CAD build for the part. Positions are in the model's coordinates, mm. Face numbers are marked on the shaded views. A direction names the side the tool comes from. Round coordinates to 2 decimals unless told otherwise and drop trailing zeros. Order: outer loops, then holes, each group sorted by start corner. A loop starts at its lowest first (then second) coordinate and runs counter-clockwise, first axis right, second up.
```python
from build123d import *

# Parameters (mm, degrees)
SKETCH_R     = 3.5
SKETCH_R_2   = 3.25
PAD_DEPTH    = 2.8
SKETCH001_R  = 4.9
PAD001_DEPTH = 5.7
PAD002_DEPTH = 11.8
SKETCH004_W  = 6.6
SKETCH004_H  = 10
PAD003_DEPTH = 6.4
SKETCH005_W  = 10
SKETCH005_H  = 6.6
SKETCH006_W  = 10
SKETCH006_H  = 5.3


with BuildPart() as part:
    # Sketch → Pad (new body)
    with BuildSketch(Plane.XZ):
        Circle(SKETCH_R)
        Circle(SKETCH_R_2, mode=Mode.SUBTRACT)
    extrude(amount=PAD_DEPTH)

    # Sketch001 (on Face4 of Pad) → Pad001 (join)
    with BuildSketch(Plane.XZ.offset(2.8)):
        Circle(SKETCH001_R)
    extrude(amount=PAD001_DEPTH)

    # Sketch002 → AdditiveLoft section 0
    with BuildSketch(Plane.XZ.offset(8.5)):
        with BuildLine():
            Line((-5.5, 2.668195), (-5.5, -2.668195))
            ThreePointArc((-5.5, -2.668195), (-4.568071, -4.918071), (-2.318195, -5.85))
            Line((-2.318195, -5.85), (2.318195, -5.85))
            ThreePointArc((2.318195, -5.85), (4.568071, -4.918071), (5.5, -2.668195))
            Line((5.5, -2.668195), (5.5, 2.668195))
            ThreePointArc((5.5, 2.668195), (4.568071, 4.918071), (2.318195, 5.85))
            Line((2.318195, 5.85), (-2.318195, 5.85))
            ThreePointArc((-2.318195, 5.85), (-4.568071, 4.918071), (-5.5, 2.668195))
        make_face()
    # Sketch003 → AdditiveLoft section 1
    with BuildSketch(Plane.XZ.offset(20.2)):
        with BuildLine():
            Line((-5.9, 7.028436), (-5.9, -7.028436))
            ThreePointArc((-5.9, -7.028436), (-5.84975, -7.14975), (-5.728436, -7.2))
            Line((-5.728436, -7.2), (5.728436, -7.2))
            ThreePointArc((5.728436, -7.2), (5.84975, -7.14975), (5.9, -7.028436))
            Line((5.9, -7.028436), (5.9, 7.028436))
            ThreePointArc((5.9, 7.028436), (5.84975, 7.14975), (5.728436, 7.2))
            Line((5.728436, 7.2), (-5.728436, 7.2))
            ThreePointArc((-5.728436, 7.2), (-5.84975, 7.14975), (-5.9, 7.028436))
        make_face()
    loft()

    # AdditiveLoft Face11 → Pad002 (add)
    with BuildSketch(Plane(origin=(0, -20.2, 0), x_dir=(-1, 0, 0), z_dir=(0, -1, 0))):
        with BuildLine():
            Line((5.9, -7.028436), (5.9, 7.028436))
            ThreePointArc((5.9, 7.028436), (5.84975, 7.14975), (5.728436, 7.2))
            Line((5.728436, 7.2), (-5.728436, 7.2))
            ThreePointArc((-5.728436, 7.2), (-5.84975, 7.14975), (-5.9, 7.028436))
            Line((-5.9, 7.028436), (-5.9, -7.028436))
            ThreePointArc((-5.9, -7.028436), (-5.84975, -7.14975), (-5.728436, -7.2))
            Line((-5.728436, -7.2), (5.728436, -7.2))
            ThreePointArc((5.728436, -7.2), (5.84975, -7.14975), (5.9, -7.028436))
        make_face()
    extrude(amount=PAD002_DEPTH)

    # Sketch004 → Pad003 (join)
    with BuildSketch(Plane.YZ.offset(-2.7)):
        with Locations((-33.5, 0)):
            Rectangle(SKETCH004_W, SKETCH004_H)
    extrude(amount=PAD003_DEPTH)

    # Sketch005 (on Face22 of Pad003) → AdditiveLoft001 section 0
    with BuildSketch(Plane(origin=(3.7, 0, 0), x_dir=(0, 0, 1), z_dir=(1, 0, 0))):
        with Locations((0, 33.5)):
            Rectangle(SKETCH005_W, SKETCH005_H)
    # Sketch006 (on Face22 of Pad003) → AdditiveLoft001 section 1
    with BuildSketch(Plane(origin=(7.7, 0, 0), x_dir=(0, 0, 1), z_dir=(1, 0, 0))):
        with Locations((0, 32.85)):
            Rectangle(SKETCH006_W, SKETCH006_H)
    loft()


solid = part.part
```
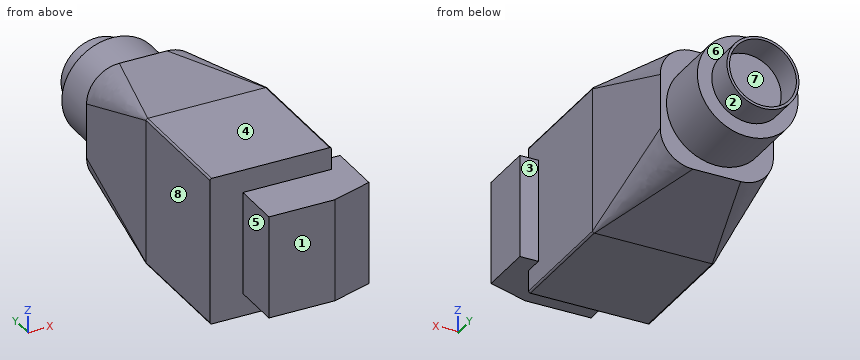
1. Mould opens along X. For the marked faces 6, 7 and 8 say: released by +X, released by -X, zero draft, split by the parting line, or undercut.
2. Cut at B-B, the plane x = 6.75. Write the cut outline in (y, z), and give its area (3 significant figures).
3. Tool access for the marked faces 1, 2, 3, 4 and 5: list every direction of +Z, -Z, +X, -X, +Y, -Y with a clear straight run to the whole face (end or side of a thin tool).
4. Drill centre lines: line 1 (Z direction, x = 0, y = -2.2); line 2 (Y direction, x = -1.25, z = 4); line 3 (X direction, y = -31, z = 6.5). Where is each one in solid material? Low to high.
5. Cut at A-A, the plane y = -21. Write the cut outline in (x, z), and give its area (3 significant figures).
6. Pin check, flat tips, straight feed: P1, Ø1, axis at x = -2.5, z = -4.5, coming from the +Y side; P2, Ø3, axis at x = -3.5, z = 5.5, coming from the +Y side; P3, Ø1, axis at y = -11.5, z = -1, coming from the -X side. Stop position of each tip, or through.
Outcome:
1. face 6: zero draft
1. face 7: undercut
1. face 8: released by -X
2. outline: (-35.81, -5) - (-30.2, -5) - (-30.2, 5) - (-35.81, 5) - close
2. area: 56.1 mm2
3. face 1: +Z, -Z, +X, -X, -Y
3. face 2: +Y
3. face 3: +Z, -Z, +X, +Y
3. face 4: +Z, +X, -X, +Y, -Y
3. face 5: +Z, -Z, -X, -Y
4. line 1: z = -3.5 to -3.25, 3.25 to 3.5
4. line 2: y = -36.8 to -2.8
4. line 3: x = -5.9 to 5.9
5. outline: (-5.9, -7.03) arc R0.17 ccw to (-5.73, -7.2) - (5.73, -7.2) arc R0.17 ccw to (5.9, -7.03) - (5.9, 7.03) arc R0.17 ccw to (5.73, 7.2) - (-5.73, 7.2) arc R0.17 ccw to (-5.9, 7.03) - close
5. area: 170 mm2
6. P1: stops at y = -2.8
6. P2: stops at y = -8.5
6. P3: stops at x = -5.62
